Print and shaded views of the part. All mm, measured from the part's lowest x, y and z. A direction names the side the tool comes from. Coordinates: 2 decimals unless noted, no trailing zeros. Loops run counter-clockwise (first coordinate to the right, second up) from the corner with the lowest first, then second, coordinate; pieces in that order, holes last. Notation, with made-up numbers: (84, 74) -> (89, 74) arc R4 ccw to (89, 80) -> close; hole circle Ø2 at (30.5, 35.25). An arc over 180 degrees is marked (long way). One line per question, with ' | ' between items. Start each with the question number.
1) Cut at C-C (x = 5.5). List the corners of the cut face in (y, z).
2) Cut at D-D (x = 12.5). List the corners of the cut face in (y, z), plus the area to 3 significant figures.
3) Drop flat-ended pins along their axis: pin 1 (7.5 mm diameter, centred on x = 8.5, y = 9.5, fed in from -Z); pin 2 (1 mm diameter, centred on x = 8.5, z = 6, fed in from +Y). Give the stop position or say it passes through.
4) Cut at A-A (y = 10). List the corners of the cut face in (x, z).
5) 3-axis set-ups, long thin cutter, end or side, ignore diameter. For the marked faces 1 and 2: which of +Z, -Z, +X, -X, +Y, -Y reach the whole face in a straight line?
6) Cut at B-B (z = 10). List the corners of the cut face in (x, y).
7) Probe L1, parallel to Y at x = 7.5, z = 20.5; L2, parallel to X at y = 0.7, z = 10; L3, parallel to Z at x = 6.5, y = 14.5. List the from-to ranges inside material, lowest first. Write a range as from..to.
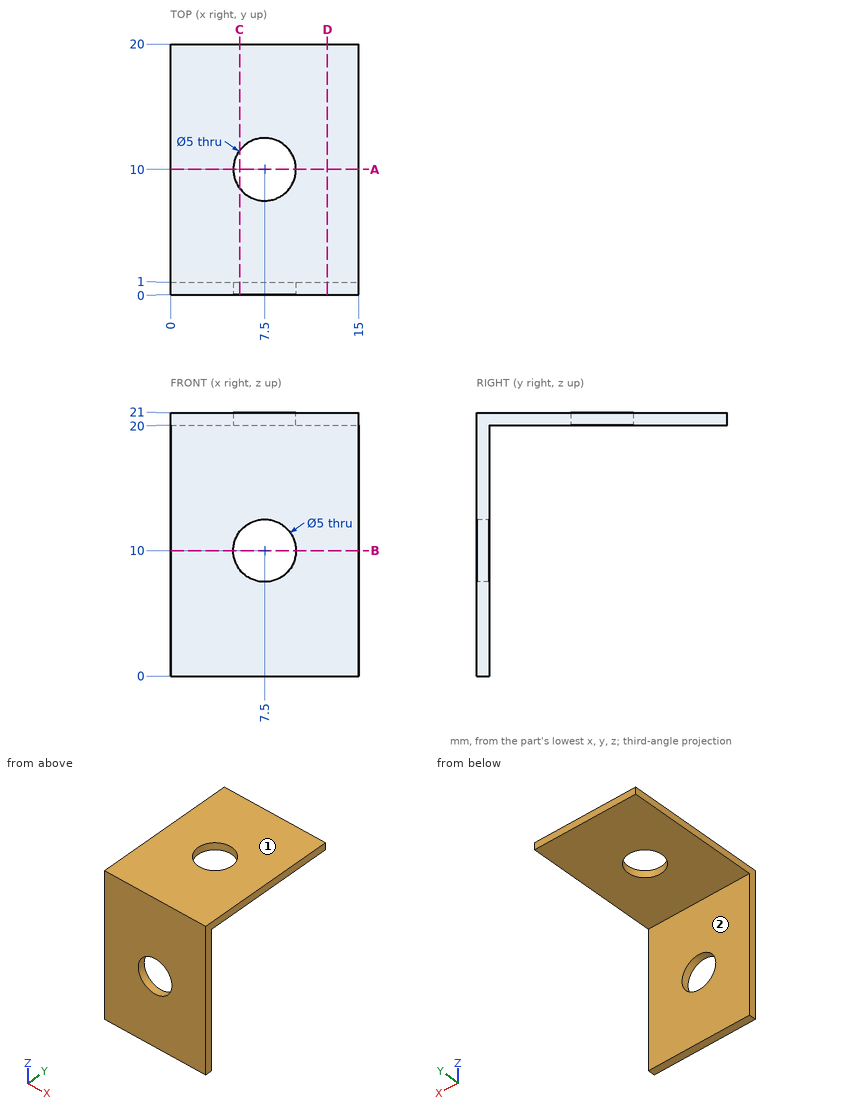
Reported:
1) outline: (0, 0) -> (1, 0) -> (1, 8.5) -> (0, 8.5) -> close; (0, 11.5) -> (1, 11.5) -> (1, 20) -> (8.5, 20) -> (8.5, 21) -> (0, 21) -> close; (11.5, 20) -> (20, 20) -> (20, 21) -> (11.5, 21) -> close
2) outline: (0, 0) -> (1, 0) -> (1, 20) -> (20, 20) -> (20, 21) -> (0, 21) -> close | area: 40.0 mm²
3) pin 1: stops at z = 20 | pin 2: stops at y = 1
4) outline: (0, 20) -> (5, 20) -> (5, 21) -> (0, 21) -> close; (10, 20) -> (15, 20) -> (15, 21) -> (10, 21) -> close
5) face 1: +Z, +X, -X, +Y, -Y | face 2: -Z, +X, -X, +Y
6) outline: (0, 0) -> (5, 0) -> (5, 1) -> (0, 1) -> close; (10, 0) -> (15, 0) -> (15, 1) -> (10, 1) -> close
7) L1: y = 0..7.5, 12.5..20 | L2: x = 0..5, 10..15 | L3: z = 20..21
